from build123d import *

# Parameters (mm, degrees)
SM_BASE_FLANGE_1_DEPTH = 375
SKETCH_6_R             = 2.5
CUT_EXTRUDE_1_DEPTH    = 10
SKETCH_7_R             = 2.5
SKETCH_7_W             = 20
SKETCH_7_H             = 30
SKETCH_7_W_2           = 3
CUT_EXTRUDE_2_DEPTH    = 3
SKETCH_8_R             = 2.5
CUT_EXTRUDE_3_DEPTH    = 1.5
SKETCH_10_W            = 100
SKETCH_10_H            = 70
CUT_EXTRUDE_5_DEPTH    = 1.5


# Sheet-metal steps are written as plain solids
with BuildPart() as part:
    # Sketch 1 → Базовая кромка1 (new, symmetric)
    with BuildSketch(Plane.XY):
        with BuildLine():
            Line((-25.25, -33), (-68.25, -33))
            ThreePointArc((-68.25, -33), (-70.371320344, -32.121320344), (-71.25, -30))
            Line((-71.25, -30), (-71.25, -3))
            ThreePointArc((-71.25, -3), (-70.371320344, -0.878679656), (-68.25, 0))
            Line((-68.25, 0), (68.25, 0))
            ThreePointArc((68.25, 0), (70.371320344, -0.878679656), (71.25, -3))
            Line((71.25, -3), (71.25, -33))
            Line((71.25, -33), (69.75, -33))
            Line((69.75, -33), (69.75, -3))
            ThreePointArc((69.75, -3), (69.310660172, -1.939339828), (68.25, -1.5))
            Line((68.25, -1.5), (-68.25, -1.5))
            ThreePointArc((-68.25, -1.5), (-69.310660172, -1.939339828), (-69.75, -3))
            Line((-69.75, -3), (-69.75, -30))
            ThreePointArc((-69.75, -30), (-69.310660172, -31.060660172), (-68.25, -31.5))
            Line((-68.25, -31.5), (-25.25, -31.5))
            Line((-25.25, -31.5), (-25.25, -33))
        make_face()
    extrude(amount=SM_BASE_FLANGE_1_DEPTH, both=True)

    # Эскиз6 → Вырез-Вытянуть1 (cut)
    with BuildSketch(Plane(origin=(71.25, 0, 0), x_dir=(0, 0, -1), z_dir=(1, 0, 0))):
        with Locations((-355, -15.5)):
            Circle(SKETCH_6_R)
        with Locations((355, -15.5)):
            Circle(SKETCH_6_R)
    extrude(amount=-CUT_EXTRUDE_1_DEPTH, mode=Mode.SUBTRACT)

    # Эскиз7 → Вырез-Вытянуть2 (cut)
    with BuildSketch(Plane.XZ.offset(33)):
        with Locations((-57.75, -325)):
            Circle(SKETCH_7_R)
        with Locations((-58.25, -360)):
            Rectangle(SKETCH_7_W, SKETCH_7_H)
        Polygon((-48.25, -375), (-25.25, -375), (-25.25, 375), (-48.25, 375), (-48.25, 345), (-48.25, -345), align=None)
        with Locations((-69.75, -360)):
            Rectangle(SKETCH_7_W_2, SKETCH_7_H)
        with Locations((-58.25, 360)):
            Rectangle(SKETCH_7_W, SKETCH_7_H)
        with Locations((-69.75, 360)):
            Rectangle(SKETCH_7_W_2, SKETCH_7_H)
        with Locations((-57.75, 325)):
            Circle(SKETCH_7_R)
    extrude(amount=-CUT_EXTRUDE_2_DEPTH, mode=Mode.SUBTRACT)

    # Эскиз8 → Вырез-Вытянуть3 (cut)
    with BuildSketch(Plane.XZ.offset(1.5)):
        with Locations((-45, -360)):
            Circle(SKETCH_8_R)
        with Locations((0, -360)):
            Circle(SKETCH_8_R)
        with Locations((45, -360)):
            Circle(SKETCH_8_R)
        with Locations(Location((45, 360, 0), (0, 0, 180))):
            Circle(SKETCH_8_R)
        with Locations(Location((0, 360, 0), (0, 0, 180))):
            Circle(SKETCH_8_R)
        with Locations(Location((-45, 360, 0), (0, 0, 180))):
            Circle(SKETCH_8_R)
    extrude(amount=-CUT_EXTRUDE_3_DEPTH, mode=Mode.SUBTRACT)

    # Эскиз10 → Вырез-Вытянуть5 (cut)
    with BuildSketch(Plane(origin=(0, 0, 0), x_dir=(1, 0, 0), z_dir=(0, 1, 0))):
        with Locations((6.75, 293.5)):
            Rectangle(SKETCH_10_W, SKETCH_10_H)
        with Locations((6.75, -293.5)):
            Rectangle(SKETCH_10_W, SKETCH_10_H)
    extrude(amount=-CUT_EXTRUDE_5_DEPTH, mode=Mode.SUBTRACT)


solid = part.part
Design review of the part built by this model. Coordinates are the model's own, in mm. A direction names the side the tool comes from. Give positions to 0.01 mm unless a question says otherwise; leave off trailing zeros. Write each loop counter-clockwise with the first axis right and the second up, starting at its lowest first coordinate (ties: lowest second). Pieces come first, ordered by that corner, then holes. Notation, with made-up numbers: M 68,8 L 92,8 A16 ccw 92,22 Z; hole C 46,6.5 d6. An arc over 180 degrees is marked long. Return JSON: item names as keys, results as strings. Group by question number.
Item 1: Take a section at B-B (x = 19). Give the boundary of the cut face in (y, z).
Item 2: Wall thickness on line 1 along Z through (x, y) = (70, -15); line 2 along Z through (x, y) = (45, -0.6); line 3 along X through (y, z) = (-4, 147): over which ranges is each line inside the solid? List them lowest first.
Item 3: Clearance check with flat-ended pins moving along their axes: pin 1 Ø12 at (x, z) = (-39.5, -289) entering from -Y; pin 2 Ø0.9 at (x, y) = (-56, -31.5) entering from +Z; pin 3 Ø0.8 at (y, z) = (-1, -287) entering from -X. State where each tip first meets the part, or that it passes through.
Item 4: Tool access review of faces 1 (the flat face through (69.75, -18, 5)), 2 (the flat face through (1, -1.5, 5)), 3 (the flat face through (71.25, -18, 5)): name each direction out of +Z, -Z, +X, -X, +Y, -Y from which nothing blocks a thin tool from reaching the whole face with its end or side.
Item 5: The part is to be moulded in two halves that separate along Y. For faces 4 (the flat face through (0, -1, 375)), 5 (the flat face through (-58, -31.5, 5)), 6 (the flat face through (-1, 0, 5)), 7 (the flat face through (-58, -33, 5)), say which applies: pulls with the +Y half, pulls with the -Y half, needs draft (parallel to the pull), parting line crosses it, or undercut.
Item 6: Take a section at A-A (z = -301). Give the boundary of the cut face in (x, y).
Item 7: Take a section at C-C (z = -5). Give the boundary of the cut face in (x, y), plus the area to 3 significant figures.
Return value:
{
 "1": {"outline": "M -1.5,-375 L 0,-375 L 0,-328.5 L -1.5,-328.5 Z; M -1.5,-258.5 L 0,-258.5 L 0,258.5 L -1.5,258.5 Z; M -1.5,328.5 L 0,328.5 L 0,375 L -1.5,375 Z"},
 "2": {"line 1": "z = -375 to -357.45, -352.55 to 352.55, 357.45 to 375", "line 2": "z = -375 to -362.5, -357.5 to -328.5, -258.5 to 258.5, 328.5 to 357.5, 362.5 to 375", "line 3": "x = -71.25 to -69.75, 69.75 to 71.25"},
 "3": {"pin 1": "stops at y = -1.5", "pin 2": "stops at z = 345", "pin 3": "stops at x = -70.79"},
 "4": {"face 1": "+Z, -Z, -Y", "face 2": "+Z, -Z", "face 3": "+Z, -Z, +X, +Y, -Y"},
 "5": {"face 4": "needs draft", "face 5": "undercut", "face 6": "pulls with the +Y half", "face 7": "pulls with the -Y half"},
 "6": {"outline": "M -71.25,-30 A3 ccw -68.25,-33 L -48.25,-33 L -48.25,-31.5 L -68.25,-31.5 A1.5 cw -69.75,-30 L -69.75,-3 A1.5 cw -68.25,-1.5 L -43.25,-1.5 L -43.25,0 L -68.25,0 A3 ccw -71.25,-3 Z; M 56.75,-1.5 L 68.25,-1.5 A1.5 cw 69.75,-3 L 69.75,-33 L 71.25,-33 L 71.25,-3 A3 ccw 68.25,0 L 56.75,0 Z"},
 "7": {"outline": "M -71.25,-30 A3 ccw -68.25,-33 L -48.25,-33 L -48.25,-31.5 L -68.25,-31.5 A1.5 cw -69.75,-30 L -69.75,-3 A1.5 cw -68.25,-1.5 L 68.25,-1.5 A1.5 cw 69.75,-3 L 69.75,-33 L 71.25,-33 L 71.25,-3 A3 ccw 68.25,0 L -68.25,0 A3 ccw -71.25,-3 Z", "area": "336 mm2"}
}
